Source: CAD feature listing. Evaluate the final solid. Frame: model axes, mm. A direction names the side the tool comes from. Round coordinates to 2 decimals unless told otherwise and drop trailing zeros. Order: outer loops, then holes, each group sorted by start corner. A loop starts at its lowest first (then second) coordinate and runs counter-clockwise, first axis right, second up. Notation, with made-up numbers: (-11, -5) - (16, -5) arc R5 cw to (16, 0) - close; hole circle Ø4 at (55, 50.25). An arc over 180 degrees is marked (long way). Return JSON: item names as keys, results as strings. Group by question number.
1) Section B-B, the plane y = 112.5. Return loops of the section in (x, z), plus the area to 3 significant figures.
2) Contact query for flat-ended pins moving along their axis: P1, Ø6, axis at y = 140, z = 174, coming from the +X side; P2, Ø0.8, axis at y = 147, z = 138.5, coming from the -X side; P3, Ø0.8, axis at y = 147, z = 174, coming from the +X side. Output: stop coordinate, or through.
3) Mould query, pull axis X, two halves, no side actions, for faces 1 (the flat face through (50, 145, 420.497)), 2 (the flat face through (11.627, 115, 207)), 3 (the cylindrical face through (87.716, 140.237, 213.192)). Classes: pulls with the +X half, pulls with the -X half, needs draft (parallel to the pull), parting line crosses it, or undercut.
4) Section A-A, the plane z = 102. Return loops of the section in (x, y), plus the area to 3 significant figures.
5) Section C-C, the plane x = 27. Return loops of the section in (y, z), plus the area to 3 significant figures.
6) Ray query, line 1 (X direction, y = 144.5, z = 364.5); line 2 (Y direction, x = 72.5, z = 87); line 3 (X direction, y = 144, z = 163). Return the intervals inside material, ascending. Write a range as from..to.
7) Access query for faces 4 (the flat face through (100, 147.856, 207)), 5 (the flat face through (50, 145, 0)), 6 (the flat face through (67, 147.856, 207)). Directions: +Z, -Z, +X, -X, +Y, -Y. A direction counts if a zero-diameter tool reaches every point of the face in a straight line with its end or side. Return the directions, or none.
Autodesk Inventor part; units mm, degrees
ref_plane "Work Plane1" through (0, -383.0536, 0) normal (0, 0, 1) x (1, 0, 0)
ref_plane "YZ Plane" through (0, 0, 0) normal (1, 0, 0) x (0, 1, 0)
ref_plane "XZ Plane" through (0, 0, 0) normal (0, 1, 0) x (-1, 0, 0)
ref_plane "Work Plane1" through (0, -383.0536, 0) normal (0, 0, 1) x (1, 0, 0)
sketch "Sketch1" plane through (0, -383.0536, 0) normal (0, 0, 1) x (1, 0, 0)
  line L0 (41.7899, 534.0845) -> (106.8774, 534.0845)
  line L1 (14.8024, 513.5226) -> (41.7899, 534.0845)
  line L2 (106.8774, 530.9095) -> (42.8616, 530.9095)
  line L3 (42.8616, 530.9095) -> (16.7266, 510.9971)
  line L4 (106.8774, 534.0845) -> (106.8774, 530.9095)
  line L5 (11.6274, 489.6345) -> (11.6274, 207.8533)
  line L6 (16.7266, 510.9971) -> (11.6274, 507.112)
  line L7 (14.8024, 513.5226) -> (8.4524, 508.6845)
  line L8 (11.6274, 489.6345) -> (11.6274, 507.112)
  line L9 (11.6274, 489.6345) -> (11.6274, 207.8533)
  line L10 (8.4524, 489.6345) -> (8.4524, 207.8533)
  line L11 (11.6274, 489.6345) -> (8.4524, 489.6345)
  line L12 (8.4524, 489.6345) -> (8.4524, 508.6845)
  point P0 (0, 383.0536)
  dimension "d0" = 3.175
extrude "Extrusion1" add sketch "Sketch1" along normal blind 420.497
sketch "Sketch2" plane through (0, -383.0536, 420.497) normal (0, 0, 1) x (1, 0, 0)
  line L0 (42.8616, 530.9095) -> (106.8774, 530.9095)
  line L1 (92.9074, 530.9095) -> (82.7474, 530.9095)
  arc A0 (82.7474, 528.3695) -> (92.9074, 528.3695) centre (87.8274, 528.3695) ccw
  line L2 (106.8774, 534.0845) -> (41.7899, 534.0845)
  arc A1 (89.5122, 530.9095) -> (86.1425, 530.9095) centre (87.8274, 528.3695) ccw
  line L3 (92.9074, 528.3695) -> (92.9074, 530.9095)
  line L4 (82.7474, 530.9095) -> (82.7474, 528.3695)
  arc A2 (83.428, 530.9095) -> (82.7474, 528.3695) centre (87.8274, 528.3695) ccw construction
  arc A3 (92.2268, 530.9095) -> (83.428, 530.9095) centre (87.8274, 528.3695) ccw
  arc A4 (92.9074, 528.3695) -> (92.2268, 530.9095) centre (87.8274, 528.3695) ccw construction
  arc A5 (86.1425, 530.9095) -> (89.5122, 530.9095) centre (87.8274, 528.3695) ccw
  line L5 (41.1835, 533.6226) -> (43.2506, 530.9095)
  line L6 (14.8024, 513.5226) -> (41.7899, 534.0845)
  arc A6 (40.1058, 528.3695) -> (50.2658, 528.3695) centre (45.1858, 528.3695) ccw
  arc A7 (43.501, 530.9095) -> (46.8707, 530.9095) centre (45.1858, 528.3695) ccw
  line L7 (50.2658, 528.3695) -> (50.2658, 530.9095)
  line L8 (11.6274, 507.112) -> (42.8616, 530.9095)
  line L9 (40.1058, 528.3695) -> (40.1058, 528.8099)
  line L10 (43.2506, 530.9095) -> (43.3386, 530.794) construction
  arc A8 (40.1264, 528.8256) -> (40.1058, 528.3695) centre (45.1858, 528.3695) ccw construction
  arc A9 (49.5853, 530.9095) -> (40.1264, 528.8256) centre (45.1858, 528.3695) ccw
  arc A10 (50.2658, 528.3695) -> (49.5853, 530.9095) centre (45.1858, 528.3695) ccw construction
  arc A11 (46.8707, 530.9095) -> (43.501, 530.9095) centre (45.1858, 528.3695) ccw
  point P0 (0, 383.0536)
  dimension "d3" = 10.16
  dimension "d4" = 13.97
  dimension "d5" = 10.16
  dimension "d8" = 6.096
  dimension "d9" = 5.715
  dimension "d10" = 3.556
  dimension "d11" = 10.16
  dimension "d12" = 6.096
  dimension "d13" = 5.715
extrude "Extrusion2" add sketch "Sketch2" against normal up to surface (420.497 mm away) contours L0 A7 L7 A6 L9 L8 | L0 A5 L3 A0 L4
properties part number "DriveBaseFront"
Geometry check:
{
 "1": {"outline": "(8.45, 0) - (11.63, 0) - (11.63, 420.5) - (8.45, 420.5) - close", "area": "1,340 mm2"},
 "2": {"P1": "x = 92.35", "P2": "x = 35.97", "P3": "x = 92.91"},
 "3": {"face 1": "needs draft", "face 2": "pulls with the +X half", "face 3": "undercut"},
 "4": {"outline": "(8.45, 106.58) - (11.63, 106.58) - (11.63, 124.06) - (16.73, 127.94) - (40.11, 145.76) - (40.11, 145.32) arc R5.08 ccw to (50.27, 145.32) - (50.27, 147.86) - (82.75, 147.86) - (82.75, 145.32) arc R5.08 ccw to (92.91, 145.32) - (92.91, 147.86) - (106.88, 147.86) - (106.88, 151.03) - (41.79, 151.03) - (14.8, 130.47) - (8.45, 125.63) - close; hole (43.5, 147.86) arc R3.05 ccw (long way) to (46.87, 147.86) - close; hole (86.14, 147.86) arc R3.05 ccw (long way) to (89.51, 147.86) - close", "area": "466 mm2"},
 "5": {"outline": "(135.77, 0) - (139.76, 0) - (139.76, 420.5) - (135.77, 420.5) - close", "area": "1,680 mm2"},
 "6": {"line 1": "33.22..38.46, 40.17..42.25, 48.12..50.2, 82.81..84.89, 90.76..92.84", "line 2": "147.86..151.03", "line 3": "32.56..37.8, 40.28..42.44, 47.94..50.09, 82.92..85.08, 90.58..92.73"},
 "7": {"face 4": "+Z, -Z, +X, -Y", "face 5": "-Z, +X, -X, +Y, -Y", "face 6": "+Z, -Z, -Y"}
}
